```python
from build123d import *

# Parameters (mm, degrees)
SKETCH008_W         = 20
SKETCH008_H         = 10
PAD052_DEPTH        = 2
SKETCH009_W         = 17.9
SKETCH009_H         = 7.9
PAD053_DEPTH        = 5
SKETCH010_W         = 16.9
SKETCH010_H         = 6.9
POCKET004_DEPTH     = 5
HOLE001_D           = 4
HOLE001_DEPTH       = 2
HOLE001_CSINK_D     = 5.5
HOLE001_CSINK_ANGLE = 90
HOLE001_TIPS_R      = 2
CHAMFER004_SIZE     = 0.3
CHAMFER005_SIZE     = 0.3
CHAMFER055_SIZE     = 0.3


with BuildPart() as part:
    # Sketch008 → Pad052 (new body)
    with BuildSketch(Plane.XZ):
        Rectangle(SKETCH008_W, SKETCH008_H)
    extrude(amount=-PAD052_DEPTH)

    # Sketch009 (on Face5 of Pad052) → Pad053 (join)
    with BuildSketch(Plane.XZ):
        Rectangle(SKETCH009_W, SKETCH009_H)
    extrude(amount=PAD053_DEPTH)

    # Sketch010 (on Face11 of Pad053) → Pocket004 (cut)
    with BuildSketch(Plane.XZ.offset(5)):
        Rectangle(SKETCH010_W, SKETCH010_H)
    extrude(amount=-POCKET004_DEPTH, mode=Mode.SUBTRACT)

    # Hole001
    with Locations(Plane(origin=(0, 2, 0), x_dir=(1, 0, 0), z_dir=(0, 1, 0))):
        with Locations((0, 0)):
            CounterSinkHole(HOLE001_D / 2, HOLE001_CSINK_D / 2, depth=HOLE001_DEPTH, counter_sink_angle=HOLE001_CSINK_ANGLE)

    # Hole001 tips → Hole001 tip 1 section 0
    with BuildSketch(Plane(origin=(0, 0, 0), x_dir=(1, 0, 0), z_dir=(0, 1, 0)), mode=Mode.PRIVATE) as hole001_tip_1_s0:
        Circle(HOLE001_TIPS_R)
    loft([hole001_tip_1_s0.sketch, Vertex(0, -1.201721, 0)], mode=Mode.SUBTRACT)

    # Chamfer004
    chamfer004_edges = [part.edges().sort_by_distance(p)[0] for p in [
        (2, 0, 0),
    ]]
    chamfer(chamfer004_edges, length=CHAMFER004_SIZE)

    # Chamfer005
    chamfer005_edges = [part.edges().sort_by_distance(p)[0] for p in [
        (0, -5, -3.95),
        (-8.95, -5, 0),
        (0, -5, 3.95),
        (8.95, -5, 0),
        (8.95, -2.5, -3.95),
        (-8.95, -2.5, -3.95),
        (8.95, -2.5, 3.95),
        (-8.95, -2.5, 3.95),
    ]]
    chamfer(chamfer005_edges, length=CHAMFER005_SIZE)

    # Chamfer055
    chamfer055_edges = [part.edges().sort_by_distance(p)[0] for p in [
        (0, 2, 5),
        (10, 2, 0),
        (0, 2, -5),
        (-10, 2, 0),
    ]]
    chamfer(chamfer055_edges, length=CHAMFER055_SIZE)


with BuildPart() as part_1:
    # Body018 placement: moved
    add(part.part.moved(Location((0, -2, -131.5))))


solid = part_1.part
```
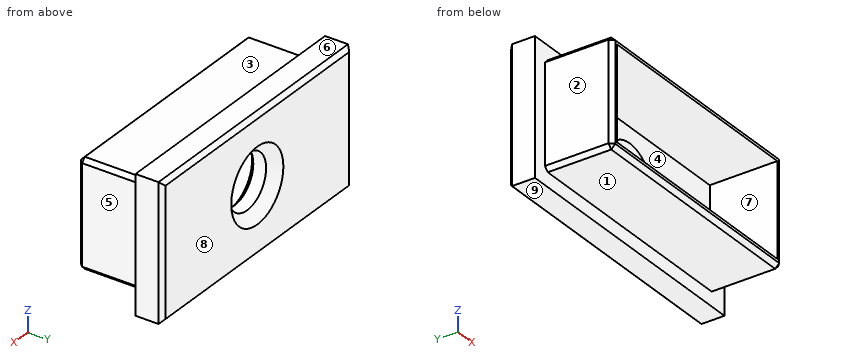
Check sheet for the modelled part. Datum: model origin and axes. Units: mm. Face numbers are marked on the shaded views. A direction names the side the tool comes from. Round coordinates to 2 decimals unless told otherwise and drop trailing zeros. Order: outer loops, then holes, each group sorted by start corner. A loop starts at its lowest first (then second) coordinate and runs counter-clockwise, first axis right, second up. Notation, with made-up numbers: (51.5, 43) -> (96.5, 43) arc R27 ccw to (96.5, 82) -> close; hole circle Ø6 at (57.25, -9.5). An arc over 180 degrees is marked (long way). One line per item, written item: value. Start each with the question number.
Q1. Cross-section at C-C (y = -2.5). Record the boundary of the cut face in (x, z), and give its area (3 significant figures).
Q2. Gauge pin test, flat ends, axial feed: pin 1 Ø1.5 at (x, y) = (1.5, -5) entering from -Z; pin 2 Ø2.5 at (y, z) = (-4, -132.5) entering from -X; pin 3 Ø1.4 at (x, y) = (2, -4) entering from +Z; pin 4 Ø2 at (x, z) = (0, -132) entering from -Y. Record the tip position at first contact, or that the pin passes through.
Q3. Cross-section at A-A (x = 0). Record the boundary of the cut face in (y, z), and give its area (3 significant figures).
Q4. Cross-section at B-B (z = -131.5). Record the boundary of the cut face in (x, y).
Q5. Set-up check for the marked faces 1, 2, 3, 4 and 5: record each of +Z, -Z, +X, -X, +Y, -Y from which the full face is reachable in a straight line by a thin tool's end or side.
Q6. Cross-section at D-D (x = 7). Record the boundary of the cut face in (y, z).
Q7. Thickness scan on line 1 (X direction, y = -1.5, z = -131.5); line 2 (X direction, y = -2.25, z = -131.5); line 3 (Z direction, x = 7.5, y = -4.25). Record the ranges inside material, lowest first.
Q8. Mould release check, pull along Z, two halves, no side actions. Record for the marked faces 6, 7, 8 and 9: pulls with the +Z half, pulls with the -Z half, needs draft (parallel to the pull), parting line crosses it, or undercut.
Completed:
1. outline: (-8.95, -135.15) -> (-8.65, -135.45) -> (8.65, -135.45) -> (8.95, -135.15) -> (8.95, -127.85) -> (8.65, -127.55) -> (-8.65, -127.55) -> (-8.95, -127.85) -> close; hole (-8.45, -134.95) -> (8.45, -134.95) -> (8.45, -128.05) -> (-8.45, -128.05) -> close
1. area: 24.6 mm²
2. pin 1: stops at z = -135.45
2. pin 2: stops at x = -8.95
2. pin 3: stops at z = -127.55
2. pin 4: passes through
3. outline: (-7, -135.15) -> (-6.7, -135.45) -> (-2, -135.45) -> (-2, -136.5) -> (-0.3, -136.5) -> (0, -136.2) -> (0, -134.25) -> (-0.75, -133.5) -> (-1.7, -133.5) -> (-2, -133.8) -> (-2, -134.95) -> (-7, -134.95) -> close; (-7, -128.05) -> (-2, -128.05) -> (-2, -129.2) -> (-1.7, -129.5) -> (-0.75, -129.5) -> (0, -128.75) -> (0, -126.8) -> (-0.3, -126.5) -> (-2, -126.5) -> (-2, -127.55) -> (-6.7, -127.55) -> (-7, -127.85) -> close
3. area: 16.2 mm²
4. outline: (-10, -2) -> (-8.95, -2) -> (-8.95, -6.7) -> (-8.65, -7) -> (-8.45, -7) -> (-8.45, -2) -> (-2.3, -2) -> (-2, -1.7) -> (-2, -0.75) -> (-2.75, 0) -> (-9.7, 0) -> (-10, -0.3) -> close; (2, -1.7) -> (2.3, -2) -> (8.45, -2) -> (8.45, -7) -> (8.65, -7) -> (8.95, -6.7) -> (8.95, -2) -> (10, -2) -> (10, -0.3) -> (9.7, 0) -> (2.75, 0) -> (2, -0.75) -> close
5. face 1: -Z, +X, -X, -Y
5. face 2: +Z, -Z, -X, -Y
5. face 3: +Z, +X, -X, -Y
5. face 4: -Y
5. face 5: +Z, -Z, +X, -Y
6. outline: (-7, -135.15) -> (-6.7, -135.45) -> (-2, -135.45) -> (-2, -136.5) -> (-0.3, -136.5) -> (0, -136.2) -> (0, -126.8) -> (-0.3, -126.5) -> (-2, -126.5) -> (-2, -127.55) -> (-6.7, -127.55) -> (-7, -127.85) -> (-7, -128.05) -> (-2, -128.05) -> (-2, -134.95) -> (-7, -134.95) -> close
7. line 1: x = -10 to -2, 2 to 10
7. line 2: x = -8.95 to -8.45, 8.45 to 8.95
7. line 3: z = -135.45 to -134.95, -128.05 to -127.55
8. face 6: pulls with the +Z half
8. face 7: undercut
8. face 8: needs draft
8. face 9: pulls with the -Z half
